```python
from build123d import *

# Parameters (mm, degrees)
IZIM1_R                     = 45
IZIM1_R_2                   = 2.45
Y_KSEKLIK_EKSTR_ZYON1_DEPTH = 20
IZIM2_R                     = 25
Y_KSEKLIK_EKSTR_ZYON2_DEPTH = 40
Y_KSEKLIK_EKSTR_ZYON3_START = -20
Y_KSEKLIK_EKSTR_ZYON3_DEPTH = 20
IZIM4_R                     = 2.5
KES_EKSTR_ZYON1_DEPTH       = 30
IZIM5_W                     = 10
IZIM5_H                     = 15
KES_EKSTR_ZYON3_DEPTH       = 30
IZIM8_R                     = 5
KES_EKSTR_ZYON4_DEPTH       = 2
IZIM10_R                    = 7.5
KES_EKSTR_ZYON5_DEPTH       = 25
IZIM12_W                    = 5
IZIM12_H                    = 18
Y_KSEKLIK_EKSTR_ZYON4_DEPTH = 30
IZIM14_W                    = 10
IZIM14_H                    = 15
KES_EKSTR_ZYON6_DEPTH       = 30
IZIM16_R                    = 15
KES_EKSTR_ZYON8_DEPTH       = 35
KES_EKSTR_ZYON9_START       = -25
KES_EKSTR_ZYON9_DEPTH       = 10
KES_EKSTR_ZYON10_START      = -15
KES_EKSTR_ZYON10_DEPTH      = 10


with BuildPart() as part:
    # Çizim1 → Yükseklik-Ekstrüzyon1 (new body)
    with BuildSketch(Plane.XY):
        Circle(IZIM1_R)
        with Locations((0, 35)):
            Circle(IZIM1_R_2, mode=Mode.SUBTRACT)
        with Locations((30.310889132, 17.5)):
            Circle(IZIM1_R_2, mode=Mode.SUBTRACT)
        with Locations((30.310889132, -17.5)):
            Circle(IZIM1_R_2, mode=Mode.SUBTRACT)
        with Locations((0, -35)):
            Circle(IZIM1_R_2, mode=Mode.SUBTRACT)
        with Locations((-30.310889132, -17.5)):
            Circle(IZIM1_R_2, mode=Mode.SUBTRACT)
        with Locations((-30.310889132, 17.5)):
            Circle(IZIM1_R_2, mode=Mode.SUBTRACT)
    extrude(amount=Y_KSEKLIK_EKSTR_ZYON1_DEPTH)

    # Çizim2 → Yükseklik-Ekstrüzyon2 (add)
    with BuildSketch(Plane(origin=(0, 0, 0), x_dir=(-1, 0, 0), z_dir=(0, 0, -1))):
        with Locations(Location((0, 0, 0), (0, 0, 180))):
            Circle(IZIM2_R)
    extrude(amount=Y_KSEKLIK_EKSTR_ZYON2_DEPTH)

    # Çizim3 → Yükseklik-Ekstrüzyon3 (add)
    with BuildSketch(Plane.XY.offset(20).offset(Y_KSEKLIK_EKSTR_ZYON3_START)):
        with BuildLine():
            Line((42.426406871, -15), (72.426406871, -15))
            Line((72.426406871, -15), (72.426406871, 15))
            Line((72.426406871, 15), (42.426406871, 15))
            ThreePointArc((42.426406871, 15), (45, 0), (42.426406871, -15))
        make_face()
        with BuildLine():
            Line((-42.426406871, -15), (-72.426406871, -15))
            Line((-72.426406871, -15), (-72.426406871, 15))
            Line((-72.426406871, 15), (-42.426406871, 15))
            ThreePointArc((-42.426406871, 15), (-45, 0), (-42.426406871, -15))
        make_face()
    extrude(amount=Y_KSEKLIK_EKSTR_ZYON3_DEPTH)

    # Çizim4 → Kes-Ekstrüzyon1 (cut)
    with BuildSketch(Plane(origin=(0, 15, 0), x_dir=(1, 0, 0), z_dir=(0, 1, 0))):
        with Locations(Location((47.426406871, -10, 0), (0, 0, 180))):
            Circle(IZIM4_R)
        with Locations((-47.426406871, -10)):
            Circle(IZIM4_R)
        with BuildLine():
            Line((72.426406871, -5), (47.426406871, -5))
            ThreePointArc((47.426406871, -5), (52.426406871, -10), (47.426406871, -15))
            Line((47.426406871, -15), (72.426406871, -15))
            Line((72.426406871, -15), (72.426406871, -5))
        make_face()
        with BuildLine():
            Line((-72.426406871, -15), (-47.426406871, -15))
            ThreePointArc((-47.426406871, -15), (-52.426406871, -10), (-47.426406871, -5))
            Line((-47.426406871, -5), (-72.426406871, -5))
            Line((-72.426406871, -5), (-72.426406871, -15))
        make_face()
    extrude(amount=-KES_EKSTR_ZYON1_DEPTH, mode=Mode.SUBTRACT)

    # Çizim5 → Kes-Ekstrüzyon3 (cut)
    with BuildSketch(Plane(origin=(72.426406871, 0, 0), x_dir=(0, 0, -1), z_dir=(1, 0, 0))):
        with Locations((-10, 0)):
            Rectangle(IZIM5_W, IZIM5_H)
    extrude(amount=-KES_EKSTR_ZYON3_DEPTH, mode=Mode.SUBTRACT)

    # Çizim8 → Kes-Ekstrüzyon4 (cut)
    with BuildSketch(Plane.XY.offset(5)):
        with Locations((64.926406871, 0)):
            Circle(IZIM8_R)
        with Locations(Location((-64.926406871, 0, 0), (0, 0, 180))):
            Circle(IZIM8_R)
    extrude(amount=-KES_EKSTR_ZYON4_DEPTH, mode=Mode.SUBTRACT)

    # Çizim10 → Kes-Ekstrüzyon5 (cut)
    with BuildSketch(Plane.XY.offset(20)):
        Circle(IZIM10_R)
    extrude(amount=-KES_EKSTR_ZYON5_DEPTH, mode=Mode.SUBTRACT)

    # Çizim12 → Yükseklik-Ekstrüzyon4 (add)
    with BuildSketch(Plane(origin=(0, 15, 0), x_dir=(1, 0, 0), z_dir=(0, 1, 0))):
        with Locations((69.926406871, 9)):
            Rectangle(IZIM12_W, IZIM12_H)
        with Locations((-69.926406871, 9)):
            Rectangle(IZIM12_W, IZIM12_H)
    extrude(amount=-Y_KSEKLIK_EKSTR_ZYON4_DEPTH)

    # Çizim14 → Kes-Ekstrüzyon6 (cut)
    with BuildSketch(Plane.ZY.offset(72.426406871)):
        with Locations((10, 0)):
            Rectangle(IZIM14_W, IZIM14_H)
    extrude(amount=-KES_EKSTR_ZYON6_DEPTH, mode=Mode.SUBTRACT)

    # Çizim16 → Kes-Ekstrüzyon8 (cut)
    with BuildSketch(Plane(origin=(0, 0, -40), x_dir=(-1, 0, 0), z_dir=(0, 0, -1))):
        Circle(IZIM16_R)
    extrude(amount=-KES_EKSTR_ZYON8_DEPTH, mode=Mode.SUBTRACT)

    # Çizim17 → Kes-Ekstrüzyon9 (cut)
    with BuildSketch(Plane(origin=(0, 0, -40), x_dir=(-1, 0, 0), z_dir=(0, 0, -1)).offset(KES_EKSTR_ZYON9_START)):
        with BuildLine():
            Line((-25, 0), (-15, 0))
            ThreePointArc((-15, 0), (-13.305162498, 6.926229199), (-8.603646545, 12.287280664))
            Line((-8.603646545, 12.287280664), (-14.339410909, 20.478801107))
            ThreePointArc((-14.339410909, 20.478801107), (-22.175270829, 11.543715331), (-25, 0))
        make_face()
    extrude(amount=-KES_EKSTR_ZYON9_DEPTH, mode=Mode.SUBTRACT)

    # Çizim18 → Kes-Ekstrüzyon10 (cut)
    with BuildSketch(Plane(origin=(0, 0, -40), x_dir=(-1, 0, 0), z_dir=(0, 0, -1)).offset(KES_EKSTR_ZYON10_START)):
        with BuildLine():
            Line((8.603646545, 12.287280664), (14.339410909, 20.478801107))
            ThreePointArc((14.339410909, 20.478801107), (22.175270829, 11.543715331), (25, 0))
            Line((25, 0), (15, 0))
            ThreePointArc((15, 0), (13.305162498, 6.926229199), (8.603646545, 12.287280664))
        make_face()
    extrude(amount=-KES_EKSTR_ZYON10_DEPTH, mode=Mode.SUBTRACT)


solid = part.part
```
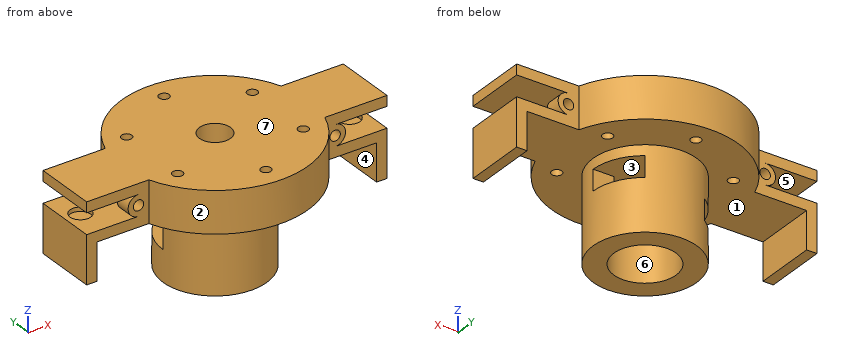
Input: part model. Units: mm. Frame: model coordinates. Face numbers are marked on the shaded views. A direction names the side the tool comes from. Coordinates: 2 decimals unless noted, no trailing zeros. Loops run counter-clockwise (first coordinate to the right, second up) from the corner with the lowest first, then second, coordinate; pieces in that order, holes last.
Q1. Section B-B, the plane y = 35. Return the cut outline in (x, z), and give its area (3 significant figures).
Results are:
outline: (-28.28, 0) - (-2.45, 0) - (-2.45, 20) - (-28.28, 20) - close; (2.45, 0) - (28.28, 0) - (28.28, 20) - (2.45, 20) - close
area: 1,030 mm2
Q2. Mould query, pull axis Z, two halves, no side actions, for the marked faces 5, 6 and 7. Classes: +Z half, -Z half, draft (parallel to the pull), parting line (faces both ways), or undercut.
Results are:
face 5: undercut
face 6: draft
face 7: +Z half
Q3. Section A-A, the plane z = -7.5. Return the cut outline in (x, y), and give its area (3 significant figures).
Results are:
outline: (-72.43, -15) - (-67.43, -15) - (-67.43, 15) - (-72.43, 15) - close; (8.6, 12.29) - (14.34, 20.48) arc R25 ccw (long way) to (25, 0) - (15, 0) arc R15 cw (long way) to start; (67.43, -15) - (72.43, -15) - (72.43, 15) - (67.43, 15) - close
area: 1,360 mm2
Q4. Section C-C, the plane y = 17.5. Return the cut outline in (x, z), and give its area (3 significant figures).
Results are:
outline: (-41.46, 0) - (-32.76, 0) - (-32.76, 20) - (-41.46, 20) - close; (-27.86, 0) - (-17.85, 0) - (-17.85, -15) - (-12.25, -15) - (-12.25, -25) - (-17.85, -25) - (-17.85, -40) - (17.85, -40) - (17.85, -15) - (12.25, -15) - (12.25, -5) - (17.85, -5) - (17.85, 0) - (27.86, 0) - (27.86, 20) - (-27.86, 20) - close; (32.76, 0) - (41.46, 0) - (41.46, 20) - (32.76, 20) - close
area: 2,780 mm2
Q5. Contact query for flat-ended pins moving along their axis: pin 1 (2.5 mm diameter, centred on x = 69, y = -0.5, fed in from -Z); pin 2 (1.5 mm diameter, centred on y = -18.5, z = 10, fed in from +X); pin 3 (6 mm diameter, centred on x = -41.5, y = -22, fed in from -Z). Output: stop coordinate, or through.
Results are:
pin 1: stops at z = -18
pin 2: stops at x = 41.35
pin 3: stops at z = 0
Q6. Section D-D, the plane z = -34. Return the cut outline in (x, y), and give its area (3 significant figures).
Results are:
outline: circle Ø50 at (0, 0); hole circle Ø30 at (0, 0)
area: 1,260 mm2
Q7. Set-up query: the marked faces 1, 2, 3 and 4. Return all of +Z, -Z, +X, -X, +Y, -Y with unobstructed straight access to the full face (end or side cutting, diameter ignored); none if empty.
Results are:
face 1: -Z
face 2: +Z, -Z, -Y
face 3: none
face 4: -Z, +Y, -Y
Q8. Line query: line 1 along X through (y, z) = (19, 10.5); line 2 along Z through (x, y) = (-21, 7); line 3 along Y through (x, z) = (-32, 6). Output: solid intervals per line, ascending.
Results are:
line 1: x = -40.79 to -32.25, -28.37 to 28.37, 32.25 to 40.79
line 2: z = -40 to -25, -15 to 20
line 3: y = -31.64 to -19.27, -15.73 to 15.73, 19.27 to 31.64
